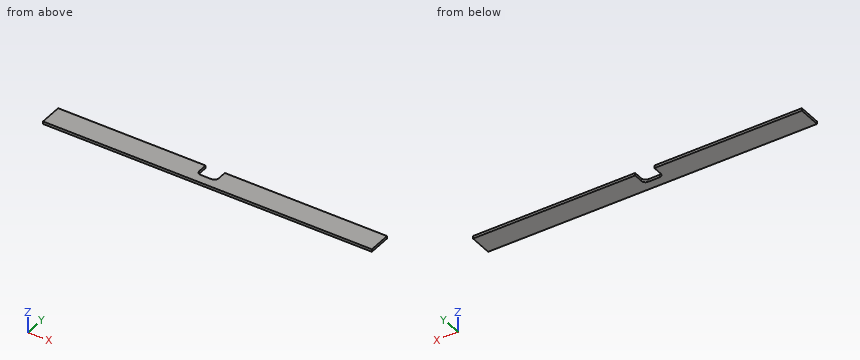
```python
from build123d import *

# Parameters (mm, degrees)
ESQUISSE1_W             = 832
ESQUISSE1_H             = 57.5
BOSS_EXTRU_1_DEPTH      = 6.5
ENL_V_MAT_EXTRU_1_DEPTH = 418.042938437


with BuildPart() as part:
    # Esquisse1 → Boss.-Extru.1 (new body)
    with BuildSketch(Plane.XY):
        Rectangle(ESQUISSE1_W, ESQUISSE1_H)
    extrude(amount=BOSS_EXTRU_1_DEPTH)

    # Esquisse2 → Enlèv. mat.-Extru.1 (cut, through all)
    with BuildSketch(Plane(origin=(0, 0, 0), x_dir=(-1, 0, 0), z_dir=(0, 0, -1))):
        with BuildLine():
            Line((4.37, -5.25), (32.84397684, -5.25))
            ThreePointArc((32.84397684, -5.25), (39.915044651, -2.321067812), (42.84397684, 4.75))
            Line((42.84397684, 4.75), (42.84397684, 32.796121721))
            ThreePointArc((42.84397684, 32.796121721), (39.915044651, 39.867189532), (32.84397684, 42.796121721))
            Line((32.84397684, 42.796121721), (4.37, 42.796121721))
            ThreePointArc((4.37, 42.796121721), (-2.701067812, 39.867189532), (-5.63, 32.796121721))
            Line((-5.63, 32.796121721), (-5.63, 4.75))
            ThreePointArc((-5.63, 4.75), (-2.701067812, -2.321067812), (4.37, -5.25))
        make_face()
    extrude(amount=-ENL_V_MAT_EXTRU_1_DEPTH, mode=Mode.SUBTRACT)


solid = part.part
```
The model under review builds one solid part; all positions refer to its coordinate system, in mm. Round coordinates to 2 decimals unless told otherwise and drop trailing zeros. Loops run counter-clockwise (first coordinate to the right, second up) from the corner with the lowest first, then second, coordinate; pieces in that order, holes last. Notation, with made-up numbers: (20, 54) - (60, 54) arc R14 cw to (60, 58) - close; hole circle Ø1 at (84, 3). An arc over 180 degrees is marked (long way). Use a Markdown table: item, result. Add a question column.
Q1. Add section A-A (z = 3.5). State the section outline as (x, y) points.
Q2. For probe 1 along X at (y, z) = (17, 2.75); probe 2 along Y at (x, z) = (-34.5, 3.75); probe 3 along Y at (x, z) = (4.5, 1.25), list the stretches that pass through material, from the lowest coordinate up.
Q3. Insertion check: pin 1 Ø3 at (x, z) = (-18, 4.5) entering from +Y. The pin has a flat end and moves straight along its axis. Give the tip position at first contact, or say it passes through.
Worked answers:
| question | item | result |
|---|---|---|
| 1 | outline | (-416, -28.75) - (416, -28.75) - (416, 28.75) - (5.63, 28.75) - (5.63, 4.75) arc R10 cw to (-4.37, -5.25) - (-32.84, -5.25) arc R10 cw to (-42.84, 4.75) - (-42.84, 28.75) - (-416, 28.75) - close |
| 2 | probe 1 | -416 to -42.84, 5.63 to 416 |
| 2 | probe 2 | -28.75 to -5.11 |
| 2 | probe 3 | -28.75 to 0.13 |
| 3 | pin 1 | y = -5.25 |
